Design review of the part built by this model. Coordinates are the model's own, in mm. Face numbers are marked on the shaded views. A direction names the side the tool comes from. Coordinates: 2 decimals unless noted, no trailing zeros. Loops run counter-clockwise (first coordinate to the right, second up) from the corner with the lowest first, then second, coordinate; pieces in that order, holes last. Notation, with made-up numbers: (60.25, 60.25) - (116.25, 60.25) arc R10 ccw to (116.25, 64.25) - close; hole circle Ø8 at (48.5, -36.75). An arc over 180 degrees is marked (long way). Return JSON: item names as keys, results as strings. Group by question number.
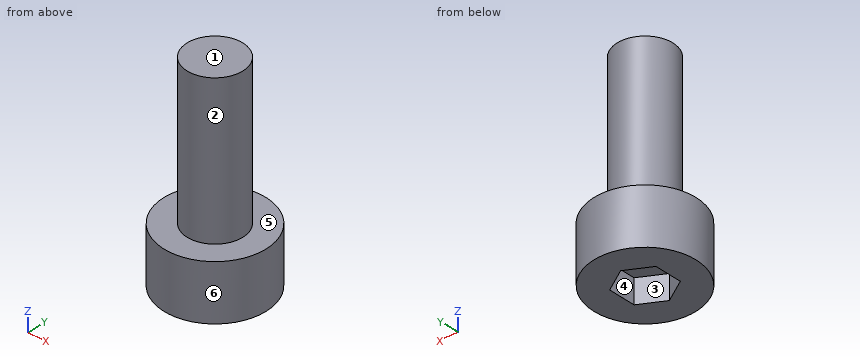
Autodesk Inventor part; units mm, degrees
ref_plane "YZ Plane" through (0, 0, 0) normal (1, 0, 0) x (0, 1, 0)
ref_plane "XZ Plane" through (0, 0, 0) normal (0, 1, 0) x (-1, 0, 0)
ref_plane "XY Plane" through (0, 0, 0) normal (0, 0, 1) x (1, 0, 0)
sketch "スケッチ1" plane through (0, 0, 0) normal (1, 0, 0) x (0, 1, 0)
  line L0 (0, 11) -> (0, 0)
  line L1 (0, 0) -> (2.75, 0)
  line L2 (2.75, 0) -> (2.75, 3)
  line L3 (2.75, 3) -> (1.5, 3)
  line L4 (1.5, 3) -> (1.5, 11)
  line L5 (1.5, 11) -> (0, 11)
  dimension "d2" = 3
  dimension "d10" = 8
  dimension "d11" = 3
  dimension "d12" = 5.5
revolve "回転1" add sketch "スケッチ1" angle 360 about axis through (0, 0, 11) along (0, 0, -1)
thread "ねじ1"
sketch "スケッチ2" plane through (0, 0, 0) normal (0, 0, -1) x (-1, 0, 0)
  line L0 (0, 1.4434) -> (1.25, 0.7217)
  line L1 (1.25, 0.7217) -> (1.25, -0.7217)
  line L2 (1.25, -0.7217) -> (0, -1.4434)
  line L3 (0, -1.4434) -> (-1.25, -0.7217)
  line L4 (-1.25, -0.7217) -> (-1.25, 0.7217)
  line L5 (-1.25, 0.7217) -> (0, 1.4434)
  circle A0 centre (0, 0) radius 2.75
  line L6 (0, 2.75) -> (0, -2.75) construction
  dimension "d7" = 2.5
extrude "押し出し1" cut sketch "スケッチ2" against normal blind 1.3 contours L0 L1 L2 L3 L4 L5
properties part number "UC-0308" material "ステンレス鋼 AISI 304"
Item 1: To check wall thickness, follow line 1 (Z direction, x = -0.5, y = -0.25); line 2 (Z direction, x = -1.8, y = 0.15); line 3 (X direction, y = 0.3, z = 0.75). State the ranges of each line that lie inside material, in increasing order. Write a range as from..to.
Item 2: Add section A-A (y = 0). State the section outline as (x, z) points.
Item 3: Add section D-D (z = 7.5). State the section outline as (x, y) points.
Item 4: Add section C-C (x = -0.95). State the section outline as (y, z) points, then the cut area to 3 significant figures.
Item 5: Add section B-B (z = 2.5). State the section outline as (x, y) points.
Item 6: Draft analysis for pull direction X (two halves, no side actions). For the marked faces 3, 4, 5 and 6, state which applies: pulls with the +X half, pulls with the -X half, needs draft (parallel to the pull), parting line crosses it, or undercut.
Item 7: For the marked faces 1 and 2, list the 3-axis set-ups (+Z, -Z, +X, -X, +Y, -Y) from which the entire face can be reached by the end or side of a thin tool; tool diameter is ignored.
Answers below:
{
 "1": {"line 1": "z = 1.3..11", "line 2": "z = 0..3", "line 3": "x = -2.73..-1.25, 1.25..2.73"},
 "2": {"outline": "(-2.75, 0) - (-1.25, 0) - (-1.25, 1.3) - (1.25, 1.3) - (1.25, 0) - (2.75, 0) - (2.75, 3) - (1.5, 3) - (1.5, 11) - (-1.5, 11) - (-1.5, 3) - (-2.75, 3) - close"},
 "3": {"outline": "circle Ø3 at (0, 0)"},
 "4": {"outline": "(-2.58, 0) - (-0.89, 0) - (-0.89, 1.3) - (0.89, 1.3) - (0.89, 0) - (2.58, 0) - (2.58, 3) - (1.16, 3) - (1.16, 11) - (-1.16, 11) - (-1.16, 3) - (-2.58, 3) - close", "area": "31.7 mm^2"},
 "5": {"outline": "circle Ø5.5 at (0, 0)"},
 "6": {"face 3": "undercut", "face 4": "undercut", "face 5": "needs draft", "face 6": "parting line crosses it"},
 "7": {"face 1": "+Z, +X, -X, +Y, -Y", "face 2": "+Z"}
}
